from build123d import *

# Parameters (mm, degrees)
F0_W     = 100
F0_H     = 100
F0_R     = 15
F1_DEPTH = 100
F2_R     = 15
F3_DEPTH = 300
F4_R     = 15
F5_DEPTH = 300
F6_R     = 15
F7_DEPTH = 300
F8_SIZE  = 8
F9_SIZE  = 5


with BuildPart() as f1:
    # F0 (on Front) → F1 (new body)
    with BuildSketch(Plane.XZ):
        with Locations((-50, -50)):
            Rectangle(F0_W, F0_H)
        with Locations((-50, -50)):
            Circle(F0_R, mode=Mode.SUBTRACT)
        with Locations((-50, -50)):
            Circle(F0_R)
    extrude(amount=-F1_DEPTH)

    # F2 (on face) → F3 (cut)
    with BuildSketch(Plane.YZ):
        with Locations((50, -50)):
            Circle(F2_R)
    extrude(amount=-F3_DEPTH, mode=Mode.SUBTRACT)

    # F4 (on face) → F5 (cut)
    with BuildSketch(Plane.XZ):
        with Locations((-50, -50)):
            Circle(F4_R)
    extrude(amount=-F5_DEPTH, mode=Mode.SUBTRACT)

    # F6 (on face) → F7 (cut)
    with BuildSketch(Plane.XY):
        with Locations((-50, 50)):
            Circle(F6_R)
    extrude(amount=-F7_DEPTH, mode=Mode.SUBTRACT)

    # F8
    f8_edges = [f1.edges().sort_by_distance(p)[0] for p in [
        (-50, 0, 0),
        (0, 0, -50),
        (-100, 0, -50),
        (-50, 0, -100),
        (-100, 50, 0),
        (-100, 100, -50),
        (-100, 50, -100),
        (0, 50, 0),
        (0, 100, -50),
        (0, 50, -100),
        (-50, 100, -100),
        (-50, 100, 0),
    ]]
    chamfer(f8_edges, length=F8_SIZE)

    # F9
    f9_edges = [f1.edges().sort_by_distance(p)[0] for p in [
        (-65, 0, -50),
        (0, 35, -50),
        (-65, 50, 0),
        (-100, 35, -50),
        (-65, 50, -100),
        (-65, 100, -50),
    ]]
    chamfer(f9_edges, length=F9_SIZE)


solid = f1.part
Source: CAD feature listing. Evaluate the final solid. Frame: model axes, mm. Give positions to 0.01 mm unless a question says otherwise; leave off trailing zeros. Order: outer loops, then holes, each group sorted by start corner. A loop starts at its lowest first (then second) coordinate and runs counter-clockwise, first axis right, second up. Notation, with made-up numbers: (79, 17.25) -> (90, 17.25) arc R15 cw to (90, 37.25) -> close; hole circle Ø1 at (9, 73). An arc over 180 degrees is marked (long way). Write item = value, one per line.
Item 1: Section query B-B (z = -50). Output: boundary loops of the cut face in (x, y), then the cut area to 3 significant figures.
Check result:
outline = (-100, 8) -> (-92, 0) -> (-70, 0) -> (-65, 5) -> (-65, 35) -> (-95, 35) -> (-100, 30) -> close; (-100, 70) -> (-95, 65) -> (-65, 65) -> (-65, 95) -> (-70, 100) -> (-92, 100) -> (-100, 92) -> close; (-35, 5) -> (-30, 0) -> (-8, 0) -> (0, 8) -> (0, 30) -> (-5, 35) -> (-35, 35) -> close; (-35, 65) -> (-5, 65) -> (0, 70) -> (0, 92) -> (-8, 100) -> (-30, 100) -> (-35, 95) -> close
area = 4,670 mm²
Item 2: Ray query, probe 1 along X at (y, z) = (50, -23); probe 2 along Y at (x, z) = (-76, -50). Return the intervals inside material, ascending.
Check result:
probe_1 = -100 to -65, -35 to 0
probe_2 = 0 to 35, 65 to 100
Item 3: Contact query for a flat-ended pin moving along its axis: pin 1 (1.5 mm diameter, centred on x = -65.5, z = -42, fed in from +Y). Output: stop coordinate, or through.
Check result:
pin_1 = 98.19
Item 4: Mould query, pull axis Y, two halves, no side actions, for faces 1 (the face through (-95.24, 58.19, -37.15)), 2 (the face through (-95, 5, -6)), 3 (the face through (-35.461, 95.243, -45.421)). Classes: +Y half, -Y half, draft (parallel to the pull), parting line (faces both ways), or undercut.
Check result:
face_1 = undercut
face_2 = -Y half
face_3 = +Y half
Item 5: Section query A-A (x = -50). Output: boundary loops of the cut face in (y, z).
Check result:
outline = (0, -92) -> (8, -100) -> (30, -100) -> (35, -95) -> (35, -65) -> (5, -65) -> (0, -70) -> close; (0, -30) -> (5, -35) -> (35, -35) -> (35, -5) -> (30, 0) -> (8, 0) -> (0, -8) -> close; (65, -95) -> (70, -100) -> (92, -100) -> (100, -92) -> (100, -70) -> (95, -65) -> (65, -65) -> close; (65, -35) -> (95, -35) -> (100, -30) -> (100, -8) -> (92, 0) -> (70, 0) -> (65, -5) -> close
Item 6: Section query D-D (y = 80). Output: boundary loops of the cut face in (x, z).
Check result:
outline = (-100, -92) -> (-92, -100) -> (-8, -100) -> (0, -92) -> (0, -8) -> (-8, 0) -> (-92, 0) -> (-100, -8) -> close; hole circle Ø30 at (-50, -50)
Item 7: Section query C-C (z = -80). Output: boundary loops of the cut face in (x, y).
Check result:
outline = (-100, 8) -> (-92, 0) -> (-8, 0) -> (0, 8) -> (0, 92) -> (-8, 100) -> (-92, 100) -> (-100, 92) -> close; hole circle Ø30 at (-50, 50)
